```python
from build123d import *

# Parameters (mm, degrees)
SKETCH_1_W          = 30
SKETCH_1_H          = 30
SKETCH_1_R          = 2
EXTRUDE_1_DEPTH     = 4
FILLET_1_R          = 5
SKETCH_2_R          = 6
EXTRUDE_2_DEPTH     = 60
SKETCH_3_R          = 3
EXTRUDE_3_DEPTH     = 16
FILLET_2_R          = 30
SKETCH_4_R          = 2.75
CUT_EXTRUDE_1_DEPTH = 3
FILLET_3_R          = 2.5
CHAMFER_4_SIZE      = 10
CHAMFER_4_SIZE2     = 3


with BuildPart() as part:
    # Эскиз1 → Бобышка-Вытянуть1 (new body)
    with BuildSketch(Plane(origin=(0, 0, 0), x_dir=(1, 0, 0), z_dir=(0, 1, 0))):
        Rectangle(SKETCH_1_W, SKETCH_1_H)
        with Locations(Location((-10, 10, 0), (0, 0, 270))):
            Circle(SKETCH_1_R, mode=Mode.SUBTRACT)
        with Locations(Location((10, 10, 0), (0, 0, 270))):
            Circle(SKETCH_1_R, mode=Mode.SUBTRACT)
        with Locations(Location((10, -10, 0), (0, 0, 270))):
            Circle(SKETCH_1_R, mode=Mode.SUBTRACT)
        with Locations(Location((-10, -10, 0), (0, 0, 270))):
            Circle(SKETCH_1_R, mode=Mode.SUBTRACT)
    extrude(amount=EXTRUDE_1_DEPTH)

    # Скругление1
    fillet_1_edges = [part.edges().sort_by_distance(p)[0] for p in [
        (15, 2, 15),
        (-15, 2, 15),
        (-15, 2, -15),
        (15, 2, -15),
    ]]
    fillet(fillet_1_edges, radius=FILLET_1_R)

    # Эскиз2 → Бобышка-Вытянуть2 (add)
    with BuildSketch(Plane(origin=(0, 4, 0), x_dir=(1, 0, 0), z_dir=(0, 1, 0))):
        with Locations(Location((0, 0, 0), (0, 0, 270))):
            Circle(SKETCH_2_R)
    extrude(amount=EXTRUDE_2_DEPTH)

    # Эскиз3 → Бобышка-Вытянуть3 (add)
    with BuildSketch(Plane(origin=(0, 64, 0), x_dir=(1, 0, 0), z_dir=(0, 1, 0))):
        with Locations(Location((0, 0, 0), (0, 0, 270))):
            Circle(SKETCH_3_R)
    extrude(amount=EXTRUDE_3_DEPTH)

    # Скругление2
    # the kernel refuses this fillet: 30 mm, written as the material it adds along each edge
    with BuildSketch(Plane(origin=(0, 64, 0), x_dir=(0, 0, 1), z_dir=(-1, 0, 0))) as fillet_2_piece_1:
        with BuildLine():
            CenterArc((33, 13.076696831), FILLET_2_R, 180, 25.841932763)
            Line((3, 13.076696831), (2.4, 13.076696831))
            Line((2.4, 13.076696831), (2.4, 0))
            Line((2.4, 0), (3, -0.6))
            ThreePointArc((3, -0.6), (4.5, -0.6), (5.46, -0.261533937))
            Line((5.46, -0.261533937), (6, 0))
        make_face()
    revolve(axis=Axis((0, 64, 0), (0, 1, 0)))

    # Эскиз4 → Вырез-Вытянуть1 (cut)
    with BuildSketch(Plane(origin=(0, 80, 0), x_dir=(1, 0, 0), z_dir=(0, 1, 0))):
        with Locations(Location((0, 0, 0), (0, 0, 270))):
            Circle(SKETCH_4_R)
    extrude(amount=-CUT_EXTRUDE_1_DEPTH, mode=Mode.SUBTRACT)

    # Скругление3
    fillet_3_edges = [part.edges().sort_by_distance(p)[0] for p in [
        (0, 77, -2.75),
    ]]
    fillet(fillet_3_edges, radius=FILLET_3_R)

    # Chamfer 4
    chamfer_4_edges = [part.edges().sort_by_distance(p)[0] for p in [
        (0, 4, -6),
    ]]
    chamfer_4_side = [part.faces().sort_by_distance(p)[0] for p in [
        (0, 34, -6),
    ]]
    chamfer(chamfer_4_edges, length=CHAMFER_4_SIZE, length2=CHAMFER_4_SIZE2, reference=chamfer_4_side[0])


solid = part.part
```
The listing builds one solid part. Answer for the finished solid, in the listing's coordinates (mm). A direction names the side the tool comes from. Coordinates: 2 decimals unless noted, no trailing zeros. Loops run counter-clockwise (first coordinate to the right, second up) from the corner with the lowest first, then second, coordinate; pieces in that order, holes last. Notation, with made-up numbers: (37.25, 77.25) -> (83.25, 77.25) arc R23 cw to (83.25, 107.25) -> close; hole circle Ø4 at (-11, 88). An arc over 180 degrees is marked (long way). Use one line per item in the form item = value. Start each with the question number.
Item 1: Consider L1, parallel to X at y = 2.2, z = 10; L2, parallel to Y at x = -2.5, z = 12.5; L3, parallel to X at y = 79.6, z = 0. Determine where each line is inside the solid, lowest interval first. Write a range as [from, to].
Item 2: A tool of negligible diameter and unlimited length cuts with its end or side. For faces 4 (the face through (0.9, 78.52, 2.86)), 5 (the face through (-15, 2, 0)), from which of +Z, -Z, +X, -X, +Y, -Y can it reach the whole face along a straight path? Write none if from no direction.
Item 3: The mould has two halves that part along Z. Classify faces 1 (the face through (12, 2, 10)), 2 (the face through (1.802, 38.65, 5.723)), 3 (the face through (0, 0, 0)): released by +Z, released by -Z, zero draft, split by the parting line, or undercut.
Item 4: The part is cut by section A-A on y = 52. Determine the outline of the cut face in (x, z), then the cut area to 3 significant figures.
Item 5: Flat-ended cylindrical pins translate along their axes: pin 1 Ø5 at (y, z) = (27.5, 2.5) entering from -X; pin 2 Ø4.5 at (x, z) = (0, 0) entering from +Y; pin 3 Ø1 at (x, y) = (8, 38.5) entering from -Z; pin 4 Ø10 at (y, z) = (44.5, 1) entering from +X. Find the tip coordinate at first contact, or state that the pin passes through.
Answer key:
q1.L1 = [-15, -12], [-8, 8], [12, 15]
q1.L2 = [0, 4]
q1.L3 = [-3, -2.75], [2.75, 3]
q2.face_4 = +Y
q2.face_5 = +Z, -Z, -X, +Y, -Y
q3.face_1 = undercut
q3.face_2 = split by the parting line
q3.face_3 = zero draft
q4.outline = circle Ø12 at (0, 0)
q4.area = 113 mm2
q5.pin_1 = -6
q5.pin_2 = 78
q5.pin_3 = through
q5.pin_4 = 6
